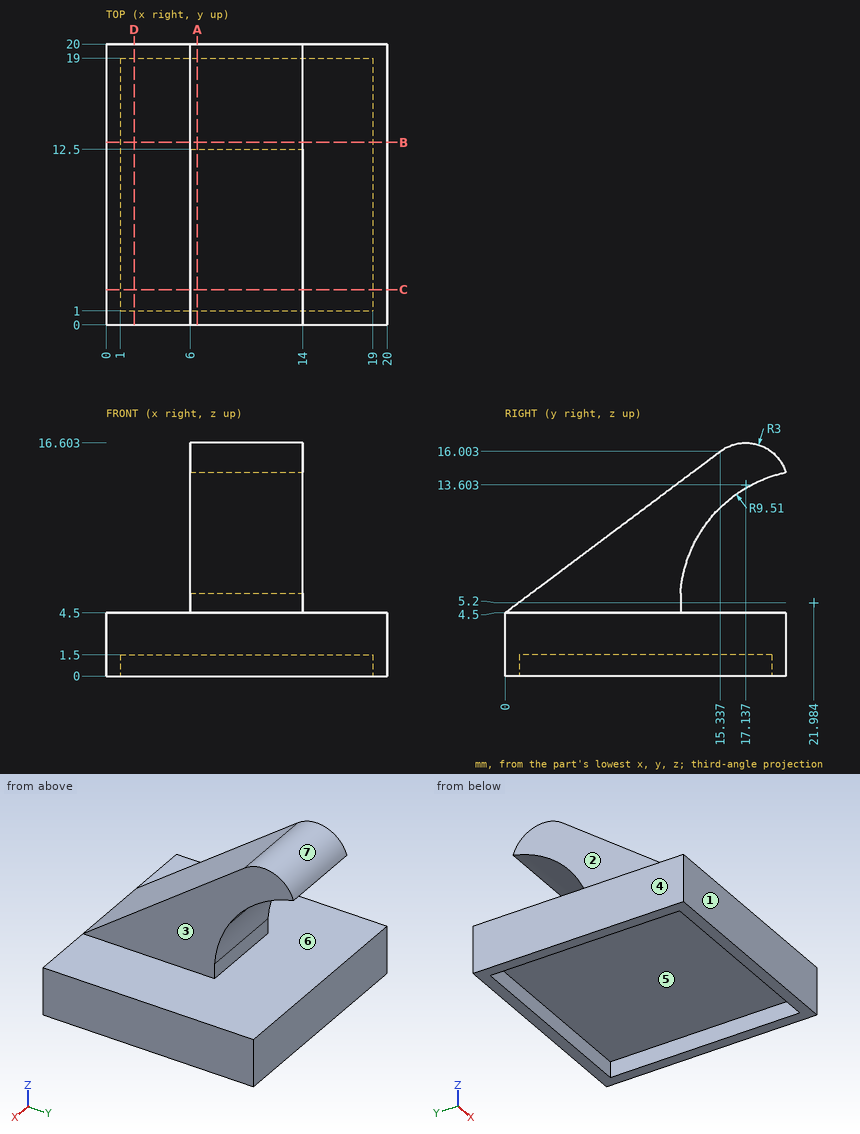
For this review, use the dimensioned drawing (mm, ordinates from the lowest corner) and the shaded views. A direction names the side the tool comes from. Round coordinates to 2 decimals unless told otherwise and drop trailing zeros. Order: outer loops, then holes, each group sorted by start corner. A loop starts at its lowest first (then second) coordinate and runs counter-clockwise, first axis right, second up.
1) For L1, parallel to X at y = 16.5, z = 1.25; L2, parallel to Z at x = 18.75, y = 16.75; L3, parallel to X at y = 14, z = 13.25, list the stretches that pass through material, from the lowest coordinate up.
The answers:
L1: x = 0 to 1, 19 to 20
L2: z = 1.5 to 4.5
L3: x = 6 to 14
2) Consider section C-C (y = 2.5). State the section outline as (x, z) points (1 decimal).
The answers:
outline: (0, 0) - (1, 0) - (1, 1.5) - (19, 1.5) - (19, 0) - (20, 0) - (20, 4.5) - (14, 4.5) - (14, 6.4) - (6, 6.4) - (6, 4.5) - (0, 4.5) - close
3) Consider section A-A (x = 6.5). State the section outline as (y, z) points, plus the area to 3 significant figures.
The answers:
outline: (0, 0) - (1, 0) - (1, 1.5) - (19, 1.5) - (19, 0) - (20, 0) - (20, 4.5) - (12.5, 4.5) - (12.5, 5.9) arc R9.51 cw to (20, 14.5) arc R3 ccw to (15.34, 16) - (0, 4.5) - close
area: 148 mm2
4) Clearance check with flat-ended pins moving along their axes: pin 1 Ø1 at (x, z) = (12.5, 7) entering from -Y (1 decimal); pin 2 Ø0.7 at (x, z) = (9, 5.5) entering from +Y; pin 3 Ø5 at (x, z) = (10.5, 12.5) entering from -Y (1 decimal). State where each tip first meets the part, or that it passes through.
The answers:
pin 1: stops at y = 2.7
pin 2: stops at y = 12.5
pin 3: stops at y = 7.3
5) Consider section D-D (x = 2). State the section outline as (y, z) points.
The answers:
outline: (0, 0) - (1, 0) - (1, 1.5) - (19, 1.5) - (19, 0) - (20, 0) - (20, 4.5) - (0, 4.5) - close
6) Draft analysis for pull direction Z (two halves, no side actions). For the marked faces 4, 5, 6 and 7, state which applies: released by +Z, released by -Z, zero draft, split by the parting line, or undercut.
The answers:
face 4: zero draft
face 5: released by -Z
face 6: undercut
face 7: released by +Z
7) Machinability: for the marked faces 1, 2 and 3, which of the approach directions +Z, -Z, +X, -X, +Y, -Y give a long, thin tool a straight path to every point of the face, cutting with its end or side? Answer none if there is none.
The answers:
face 1: +Z, -Z, +X, -X, -Y
face 2: +Z, -X, +Y, -Y
face 3: +Z, +X, +Y, -Y
8) Consider section B-B (y = 13). State the section outline as (x, z) points.
The answers:
outline: (0, 0) - (1, 0) - (1, 1.5) - (19, 1.5) - (19, 0) - (20, 0) - (20, 4.5) - (0, 4.5) - close; (6, 8.32) - (14, 8.32) - (14, 14.25) - (6, 14.25) - close
